Read the model definition and answer for the solid it produces. Units are mm, in the model's axes. A direction names the side the tool comes from. Coordinates: 2 decimals unless noted, no trailing zeros. Order: outer loops, then holes, each group sorted by start corner. A loop starts at its lowest first (then second) coordinate and runs counter-clockwise, first axis right, second up. Notation, with made-up numbers: (70.25, 53.5) -> (100.25, 53.5) arc R22 ccw to (100.25, 90.5) -> close; hole circle Ø7 at (29.25, 80.5). An arc over 180 degrees is marked (long way). Answer as a JSON object with one key per item and string values. Group by question number.
1) Section C-C on x = -73.5 is taken. Determine the outline of the cut face in (y, z).
2) Consider L1, parallel to Z at x = -107, y = -0.75; L2, parallel to Z at x = -104, y = -1.7; L3, parallel to Z at x = -111, y = -1.6. Determine where each line is inside the solid, lowest interval first.
3) A tool of negligible diameter and unlimited length cuts with its end or side. For faces 4 (the cylindrical face through (-59.737, -1.503, -28.463)), 5 (the flat face through (-93.63, -1.5, -0.49)), from which of +Z, -Z, +X, -X, +Y, -Y can it reach the whole face along a straight path? Write none if from no direction.
4) Given pin 1 (1 mm diameter, centred on x = -97.5, z = -10.5, fed in from +Y), flat-ended and moving along its own axis, determine where the tip first touches the part or whether it passes through.
5) Section B-B on z = -14 is taken. Determine the outline of the cut face in (x, y).
6) Determine the mould class of faces 1 (the flat face through (-94.22, -1.5, 49.21)), 2 (the cylindrical face through (-109.916, -1.503, 61.499)), 3 (the flat face through (-119.226, -1.503, -4.865)) for opening direction X: released by +X, released by -X, zero draft, split by the parting line, or undercut.
7) Section A-A on y = -1.2 is taken. Count the separate pieces of the cut face and the enclosed holes in it, and give its area (3 significant figures).
from build123d import *

# Parameters (mm, degrees)
F0_R     = 3.175
F1_DEPTH = 3.048


with BuildPart() as f1:
    # F0 (on Front) → F1 (new body)
    with BuildSketch(Plane.XZ):
        with BuildLine():
            ThreePointArc((-97.190643335, 74.3602226092), (-100.121969827, 80.8210350642), (-106.7062930619, 83.463280344))
            Line((-106.7062930619, 83.463280344), (-106.7062930619, 77.113280344))
            ThreePointArc((-106.7062930619, 77.113280344), (-104.4612290316, 76.1833443743), (-103.5312930619, 73.938280344))
            ThreePointArc((-103.5312930619, 73.938280344), (-104.4612290316, 71.6932163137), (-106.7062930619, 70.763280344))
            Line((-106.7062930619, 70.763280344), (-106.7062930619, 64.413280344))
            ThreePointArc((-106.7062930619, 64.413280344), (-99.9711009711, 67.2030882532), (-97.1812930619, 73.938280344))
            ThreePointArc((-97.1812930619, 73.938280344), (-97.1836309171, 74.1493032709), (-97.190643335, 74.3602226092))
        make_face()
        with BuildLine():
            Line((-106.7062930619, 77.113280344), (-106.7062930619, 83.463280344))
            ThreePointArc((-106.7062930619, 83.463280344), (-113.3589155182, 80.7550419985), (-116.2284645394, 74.1703909904))
            ThreePointArc((-116.2284645394, 74.1703909904), (-113.5230547163, 67.2856578877), (-106.7062930619, 64.413280344))
            Line((-106.7062930619, 64.413280344), (-106.7062930619, 70.763280344))
            ThreePointArc((-106.7062930619, 70.763280344), (-109.8812930619, 73.938280344), (-106.7062930619, 77.113280344))
        make_face()
        with BuildLine():
            Line((-91.3305569208, 24.7476115825), (-97.190643335, 74.3602226092))
            ThreePointArc((-97.190643335, 74.3602226092), (-97.1836309171, 74.1493032709), (-97.1812930619, 73.938280344))
            ThreePointArc((-97.1812930619, 73.938280344), (-99.9711009711, 67.2030882532), (-106.7062930619, 64.413280344))
            Line((-106.7062930619, 64.413280344), (-106.7062930619, 36.6726289093))
            ThreePointArc((-106.7062930619, 36.6726289093), (-96.977221933, 33.3419822194), (-91.3305569208, 24.7476115825))
        make_face()
        with BuildLine():
            ThreePointArc((-106.7062930619, 64.413280344), (-113.5230547163, 67.2856578877), (-116.2284645394, 74.1703909904))
            Line((-116.2284645394, 74.1703909904), (-121.9364228074, 25.2763310577))
            ThreePointArc((-121.9364228074, 25.2763310577), (-116.2172401334, 33.5081564674), (-106.7062930619, 36.6726289093))
            Line((-106.7062930619, 36.6726289093), (-106.7062930619, 64.413280344))
        make_face()
        with Locations((-112.9446998239, 60.5451092124)):
            Circle(F0_R, mode=Mode.SUBTRACT)
        with BuildLine():
            Line((-90.8334058763, 20.5386358703), (-91.3305569208, 24.7476115825))
            ThreePointArc((-91.3305569208, 24.7476115825), (-96.977221933, 33.3419822194), (-106.7062930619, 36.6726289093))
            Line((-106.7062930619, 36.6726289093), (-106.7062930619, 23.9726289093))
            ThreePointArc((-106.7062930619, 23.9726289093), (-104.4612290316, 23.0426929396), (-103.5312930619, 20.7976289093))
            ThreePointArc((-103.5312930619, 20.7976289093), (-104.4612290316, 18.5525648791), (-106.7062930619, 17.6226289093))
            Line((-106.7062930619, 17.6226289093), (-106.7062930619, 4.9226289093))
            ThreePointArc((-106.7062930619, 4.9226289093), (-96.9573127505, 8.2687419721), (-91.3180887059, 16.8965019314))
            Line((-91.3180887059, 16.8965019314), (-90.8334058763, 20.5386358703))
        make_face()
        with BuildLine():
            ThreePointArc((-90.8312930619, 20.7976289093), (-90.9566036008, 22.7883340306), (-91.3305569208, 24.7476115825))
            Line((-91.3305569208, 24.7476115825), (-90.8334058763, 20.5386358703))
            ThreePointArc((-90.8334058763, 20.5386358703), (-90.8318212743, 20.6681280809), (-90.8312930619, 20.7976289093))
        make_face()
        with BuildLine():
            Line((-122.5585151056, 19.9475222821), (-121.9364228074, 25.2763310577))
            ThreePointArc((-121.9364228074, 25.2763310577), (-122.4742098212, 22.6383967032), (-122.5585151056, 19.9475222821))
        make_face()
        with BuildLine():
            ThreePointArc((-106.7062930619, 36.6726289093), (-116.2172401334, 33.5081564674), (-121.9364228074, 25.2763310577))
            Line((-121.9364228074, 25.2763310577), (-122.5585151056, 19.9475222821))
            Line((-122.5585151056, 19.9475222821), (-122.2211590079, 17.435403504))
            ThreePointArc((-122.2211590079, 17.435403504), (-116.6722425071, 8.4406277903), (-106.7062930619, 4.9226289093))
            Line((-106.7062930619, 4.9226289093), (-106.7062930619, 17.6226289093))
            ThreePointArc((-106.7062930619, 17.6226289093), (-109.8812930619, 20.7976289093), (-106.7062930619, 23.9726289093))
            Line((-106.7062930619, 23.9726289093), (-106.7062930619, 36.6726289093))
        make_face()
        with BuildLine():
            ThreePointArc((-91.3180887059, 16.8965019314), (-90.9700213942, 18.7034992571), (-90.8334058763, 20.5386358703))
            Line((-90.8334058763, 20.5386358703), (-91.3180887059, 16.8965019314))
        make_face()
        with BuildLine():
            Line((-122.2211590079, 17.435403504), (-122.5585151056, 19.9475222821))
            ThreePointArc((-122.5585151056, 19.9475222821), (-122.4400541325, 18.6847191686), (-122.2211590079, 17.435403504))
        make_face()
        with BuildLine():
            Line((-95.8810541015, -17.3917585872), (-91.3180887059, 16.8965019314))
            ThreePointArc((-91.3180887059, 16.8965019314), (-96.9573127505, 8.2687419721), (-106.7062930619, 4.9226289093))
            Line((-106.7062930619, 4.9226289093), (-106.7062930619, -17.0063675549))
            ThreePointArc((-106.7062930619, -17.0063675549), (-106.3674067324, -17.0123980174), (-106.028949514, -17.0304817689))
            Line((-106.028949514, -17.0304817689), (-95.8810541015, -17.3917585872))
        make_face()
        with BuildLine():
            ThreePointArc((-106.7062930619, 4.9226289093), (-116.6722425071, 8.4406277903), (-122.2211590079, 17.435403504))
            Line((-122.2211590079, 17.435403504), (-116.1465497043, -27.7991133993))
            ThreePointArc((-116.1465497043, -27.7991133993), (-113.8757039222, -20.2603889298), (-106.7062930619, -17.0063675549))
            Line((-106.7062930619, -17.0063675549), (-106.7062930619, 4.9226289093))
        make_face()
        with BuildLine():
            Line((-61.9738877873, -18.5988929403), (-95.8810541015, -17.3917585872))
            Line((-95.8810541015, -17.3917585872), (-97.0973222591, -26.5313675549))
            Line((-97.0973222591, -26.5313675549), (-70.1937930619, -26.5313675549))
            ThreePointArc((-70.1937930619, -26.5313675549), (-67.7682035466, -20.819734771), (-61.9738877873, -18.5988929403))
        make_face()
        with BuildLine():
            Line((-97.0973222591, -26.5313675549), (-95.8810541015, -17.3917585872))
            Line((-95.8810541015, -17.3917585872), (-106.028949514, -17.0304817689))
            ThreePointArc((-106.028949514, -17.0304817689), (-99.7357363304, -20.0400684666), (-97.1812930619, -26.5313675549))
            Line((-97.1812930619, -26.5313675549), (-97.0973222591, -26.5313675549))
        make_face()
        with BuildLine():
            ThreePointArc((-106.7062930619, -17.0063675549), (-113.8757039222, -20.2603889298), (-116.1465497043, -27.7991133993))
            ThreePointArc((-116.1465497043, -27.7991133993), (-112.8850424708, -33.78041444), (-106.4626122264, -36.053249966))
            Line((-106.4626122264, -36.053249966), (-106.269860848, -36.0463637148))
            ThreePointArc((-106.269860848, -36.0463637148), (-99.8185270294, -33.1104483479), (-97.1812930619, -26.5313675549))
            Line((-97.1812930619, -26.5313675549), (-103.5312930619, -26.5313675549))
            ThreePointArc((-103.5312930619, -26.5313675549), (-108.9513570922, -28.7764315852), (-106.7062930619, -23.3563675549))
            Line((-106.7062930619, -23.3563675549), (-106.7062930619, -17.0063675549))
        make_face()
        with BuildLine():
            Line((-70.1937930619, -26.5313675549), (-97.0973222591, -26.5313675549))
            Line((-97.0973222591, -26.5313675549), (-97.1812930619, -26.5313675549))
            ThreePointArc((-97.1812930619, -26.5313675549), (-99.8185270294, -33.1104483479), (-106.269860848, -36.0463637148))
            Line((-106.269860848, -36.0463637148), (-61.9728980991, -34.4638068736))
            ThreePointArc((-61.9728980991, -34.4638068736), (-67.7678472317, -32.2433441728), (-70.1937930619, -26.5313675549))
        make_face()
        with BuildLine():
            ThreePointArc((-54.3187930619, -26.5313675549), (-56.544660278, -21.0194570702), (-61.9738877873, -18.5988929403))
            ThreePointArc((-61.9738877873, -18.5988929403), (-67.7682035466, -20.819734771), (-70.1937930619, -26.5313675549))
            ThreePointArc((-70.1937930619, -26.5313675549), (-67.7678472317, -32.2433441728), (-61.9728980991, -34.4638068736))
            ThreePointArc((-61.9728980991, -34.4638068736), (-56.544316444, -32.0429217247), (-54.3187930619, -26.5313675549))
        make_face()
        with BuildLine():
            ThreePointArc((-59.0812930619, -26.5313675549), (-62.2562930619, -29.7063675549), (-65.4312930619, -26.5313675549))
            ThreePointArc((-65.4312930619, -26.5313675549), (-62.2562930619, -23.3563675549), (-59.0812930619, -26.5313675549))
        make_face(mode=Mode.SUBTRACT)
        with BuildLine():
            Line((-106.269860848, -36.0463637148), (-106.4626122264, -36.053249966))
            ThreePointArc((-106.4626122264, -36.053249966), (-106.3662191065, -36.0502947373), (-106.269860848, -36.0463637148))
        make_face()
        with BuildLine():
            Line((-106.028949514, -17.0304817689), (-106.7062930619, -17.0063675549))
            Line((-106.7062930619, -17.0063675549), (-106.7062930619, -23.3563675549))
            ThreePointArc((-106.7062930619, -23.3563675549), (-104.4612290316, -24.2863035246), (-103.5312930619, -26.5313675549))
            Line((-103.5312930619, -26.5313675549), (-97.1812930619, -26.5313675549))
            ThreePointArc((-97.1812930619, -26.5313675549), (-99.7357363304, -20.0400684666), (-106.028949514, -17.0304817689))
        make_face()
    extrude(amount=F1_DEPTH)


solid = f1.part
Worked answers:
{
 "1": {"outline": "(-3.05, -34.88) -> (0, -34.88) -> (0, -18.19) -> (-3.05, -18.19) -> close"},
 "2": {"L1": "z = -36.05 to -29.69, -23.37 to 17.64, 23.96 to 70.78, 77.1 to 83.46", "L2": "z = -35.97 to -28.19, -24.87 to 19.14, 22.46 to 72.28, 75.6 to 83.07", "L3": "z = -35.03 to 58.04, 63.05 to 82.44"},
 "3": {"face 4": "+Y, -Y", "face 5": "+X, +Y, -Y"},
 "4": {"pin 1": "stops at y = 0"},
 "5": {"outline": "(-118, -3.05) -> (-95.43, -3.05) -> (-95.43, 0) -> (-118, 0) -> close"},
 "6": {"face 1": "released by +X", "face 2": "undercut", "face 3": "released by -X"},
 "7": {"separate pieces": "1", "enclosed holes": "6", "area": "3,390 mm²"}
}
